Check sheet for the modelled part. Datum: model origin and axes. Units: mm. Face numbers are marked on the shaded views. A direction names the side the tool comes from. Give positions to 0.01 mm unless a question says otherwise; leave off trailing zeros. Loops run counter-clockwise (first coordinate to the right, second up) from the corner with the lowest first, then second, coordinate; pieces in that order, holes last. Notation, with made-up numbers: (73.5, 71) - (112.5, 71) arc R25 ccw to (112.5, 91) - close; hole circle Ø5 at (55.25, 19.5). An arc over 180 degrees is marked (long way). Use CSV: the item, a comma, the result in double quotes.
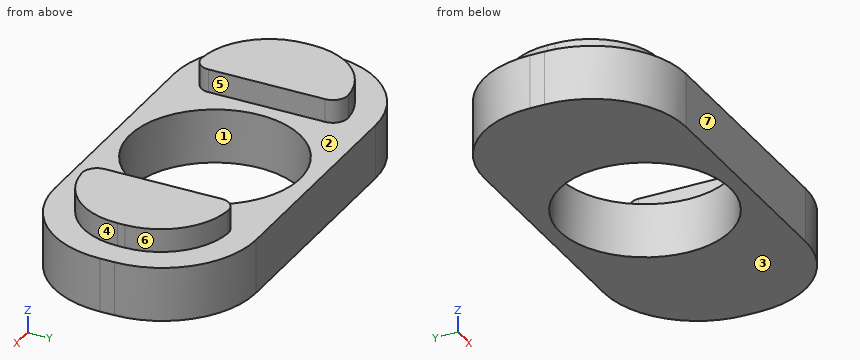
from build123d import *

# Parameters (mm, degrees)
F0_W     = 54
F0_H     = 26
F0_R     = 11
F1_DEPTH = 7
F2_R     = 12.0710678119
F3_W     = 10.4644660941
F3_H     = 18.9284660941
F4_DEPTH = 3
F5_R     = 9
F6_DEPTH = 3
F7_R     = 9
F8_R     = 1.9313708499


with BuildPart() as f1:
    # F0 (on Top) → F1 (new body)
    with BuildSketch(Plane.XY):
        Rectangle(F0_W, F0_H)
        Circle(F0_R, mode=Mode.SUBTRACT)
    extrude(amount=F1_DEPTH)

    # F2
    f2_edges = [f1.edges().sort_by_distance(p)[0] for p in [
        (-27, -13, 3.5),
        (-27, 13, 3.5),
        (27, -13, 3.5),
        (27, 13, 3.5),
    ]]
    fillet(f2_edges, radius=F2_R)

    # F3 (on face) → F4 (join)
    with BuildSketch(Plane.XY.offset(7)):
        with Locations((-18.232233047, 0.000233047)):
            Rectangle(F3_W, F3_H)
        with Locations((18.232233047, 0.000233047)):
            Rectangle(F3_W, F3_H)
    extrude(amount=F4_DEPTH)

    # F5
    f5_edges = [f1.edges().sort_by_distance(p)[0] for p in [
        (-23.464466, -9.464, 8.5),
        (23.464466, -9.464, 8.5),
        (-23.464466, 9.464466, 8.5),
        (23.464466, 9.464466, 8.5),
    ]]
    fillet(f5_edges, radius=F5_R)

    # F3 (on face) → F6 (join)
    with BuildSketch(Plane.XY.offset(7)):
        with Locations((-18.232233047, 0.000233047)):
            Rectangle(F3_W, F3_H)
        with Locations((18.232233047, 0.000233047)):
            Rectangle(F3_W, F3_H)
    extrude(amount=F6_DEPTH)

    # F7
    f7_edges = [f1.edges().sort_by_distance(p)[0] for p in [
        (-23.464466, 9.464466, 8.5),
        (-23.464466, -9.464, 8.5),
        (23.464466, -9.464, 8.5),
        (23.464466, 9.464466, 8.5),
    ]]
    fillet(f7_edges, radius=F7_R)

    # F8
    f8_edges = [f1.edges().sort_by_distance(p)[0] for p in [
        (13, -9.464, 8.5),
        (13, 9.464466, 8.5),
        (-13, -9.464, 8.5),
        (-13, 9.464466, 8.5),
    ]]
    fillet(f8_edges, radius=F8_R)


solid = f1.part
1. Go/stop test with flat-tipped pins: pin 1 Ø3.5 at (y, z) = (-0.5, 9) entering from +X; pin 2 Ø1.5 at (y, z) = (8.5, 7.5) entering from +X; pin 3 Ø1 at (x, z) = (-19.5, 5) entering from +Y. Record where each tip stops, or that it passes through.
Completed:
pin 1,"stops at x = 23.46"
pin 2,"stops at x = 24.75"
pin 3,"stops at y = 12.29"
2. Scan lines: line 1 along Y through (x, z) = (0, 4); line 2 along Z through (x, y) = (9, -8.25); line 3 along X through (y, z) = (-4.25, 4.5). Record each from-to range of solid material in increasing order.
Completed:
line 1,"y = -13 to -11, 11 to 13"
line 2,"z = 0 to 7"
line 3,"x = -26.53 to -10.15, 10.15 to 26.53"
3. Sectioned sample at A-A, the plane x = 0. Record the boundary of the cut face in (y, z), and give its area (3 significant figures).
Completed:
outline,"(-13, 0) - (-11, 0) - (-11, 7) - (-13, 7) - close; (11, 0) - (13, 0) - (13, 7) - (11, 7) - close"
area,"28.0 mm²"
4. Set-up check for the marked faces 5, 6 and 7: record each of +Z, -Z, +X, -X, +Y, -Y from which the full face is reachable in a straight line by a thin tool's end or side.
Completed:
face 5,"+Z, +Y, -Y"
face 6,"+Z, +X, +Y"
face 7,"+Z, -Z, +X, -X, -Y"
5. Sectioned sample at B-B, the plane y = -5.25. Record the boundary of the cut face in (x, z), and give its area (3 significant figures).
Completed:
outline,"(-26.2, 0) - (-9.67, 0) - (-9.67, 7) - (-13, 7) - (-13, 10) - (-22.09, 10) - (-22.09, 7) - (-26.2, 7) - close; (9.67, 0) - (26.2, 0) - (26.2, 7) - (22.09, 7) - (22.09, 10) - (13, 10) - (13, 7) - (9.67, 7) - close"
area,"286 mm²"
6. Release check for a two-part mould opening along X. For the marked faces 1, 2, 3 and 4 record: released by +X, released by -X, zero draft, split by the parting line, or undercut.
Completed:
face 1,"undercut"
face 2,"undercut"
face 3,"zero draft"
face 4,"released by +X"
7. Sectioned sample at D-D, the plane x = -19.5. Record the boundary of the cut face in (y, z).
Completed:
outline,"(-12.1, 0) - (12.1, 0) - (12.1, 7) - (7.92, 7) - (7.92, 10) - (-7.92, 10) - (-7.92, 7) - (-12.1, 7) - close"
8. Sectioned sample at C-C, the plane z = 3. Record the boundary of the cut face in (x, y), and give its area (3 significant figures).
Completed:
outline,"(-27, -0.93) arc R12.07 ccw to (-14.93, -13) - (14.93, -13) arc R12.07 ccw to (27, -0.93) - (27, 0.93) arc R12.07 ccw to (14.93, 13) - (-14.93, 13) arc R12.07 ccw to (-27, 0.93) - close; hole circle Ø22 at (0, 0)"
area,"899 mm²"
